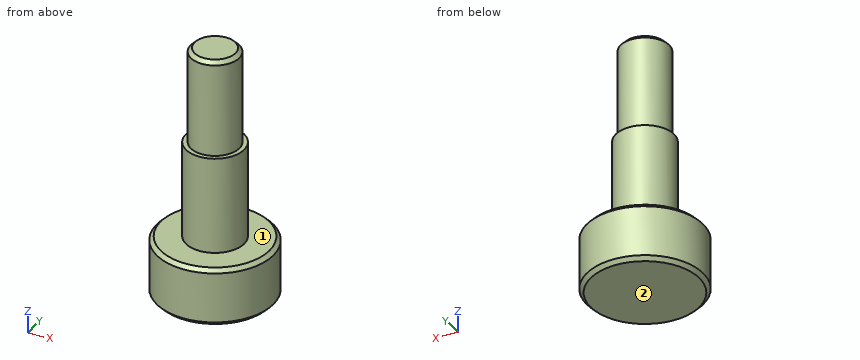
```python
from build123d import *

# Parameters (mm, degrees)
SKETCH_1_R      = 3
EXTRUDE_1_DEPTH = 3
SKETCH_2_R      = 1.5
EXTRUDE_2_DEPTH = 5
SKETCH_3_R      = 1.25
EXTRUDE_3_DEPTH = 5
CHAMFER_1_SIZE  = 0.2


with BuildPart() as part:
    # 草图1 → 凸台-拉伸1 (new body)
    with BuildSketch(Plane.XY):
        Circle(SKETCH_1_R)
    extrude(amount=EXTRUDE_1_DEPTH)

    # 草图2 → 凸台-拉伸2 (add)
    with BuildSketch(Plane.XY.offset(3)):
        Circle(SKETCH_2_R)
    extrude(amount=EXTRUDE_2_DEPTH)

    # 草图3 → 凸台-拉伸3 (add)
    with BuildSketch(Plane.XY.offset(8)):
        Circle(SKETCH_3_R)
    extrude(amount=EXTRUDE_3_DEPTH)

    # 倒角1
    chamfer_1_edges = [part.edges().sort_by_distance(p)[0] for p in [
        (-1.25, 0, 13),
        (-3, 0, 0),
        (-3, 0, 3),
    ]]
    chamfer(chamfer_1_edges, length=CHAMFER_1_SIZE)


solid = part.part
```
Input: part model. Units: mm. Frame: model coordinates. Face numbers are marked on the shaded views. A direction names the side the tool comes from. Give positions to 0.01 mm unless a question says otherwise; leave off trailing zeros. Order: outer loops, then holes, each group sorted by start corner. A loop starts at its lowest first (then second) coordinate and runs counter-clockwise, first axis right, second up.
1. Set-up query: the marked faces 1 and 2. Return all of +Z, -Z, +X, -X, +Y, -Y with unobstructed straight access to the full face (end or side cutting, diameter ignored); none if empty.
Computed:
face 1: +Z
face 2: -Z, +X, -X, +Y, -Y
2. Line query: probe 1 along Z at (x, y) = (-1.7, 1.4); probe 2 along Z at (x, y) = (-0.4, -1.35); probe 3 along Y at (x, z) = (-0.05, 4.25). Output: solid intervals per line, ascending.
Computed:
probe 1: z = 0 to 3
probe 2: z = 0 to 8
probe 3: y = -1.5 to 1.5
3. Pin query (flat end, axial travel): pin 1 Ø3 at (x, z) = (1, 9) entering from -Y; pin 2 Ø1 at (x, y) = (-1, 2) entering from +Z; pin 3 Ø2 at (x, z) = (-2, 3.5) entering from -Y. Return the tip coordinate at first contact, or that it passes through.
Computed:
pin 1: stops at y = -1.5
pin 2: stops at z = 3
pin 3: stops at y = -2.71
4. Cut plane D-D (z = 10.75). Return loops of the section in (x, y), and give its area (3 significant figures).
Computed:
outline: circle Ø2.5 at (0, 0)
area: 4.91 mm2
5. Cut plane A-A (x = 0). Return loops of the section in (y, z), and give its area (3 significant figures).
Computed:
outline: (-3, 0.2) - (-2.8, 0) - (2.8, 0) - (3, 0.2) - (3, 2.8) - (2.8, 3) - (1.5, 3) - (1.5, 8) - (1.25, 8) - (1.25, 12.8) - (1.05, 13) - (-1.05, 13) - (-1.25, 12.8) - (-1.25, 8) - (-1.5, 8) - (-1.5, 3) - (-2.8, 3) - (-3, 2.8) - close
area: 45.4 mm2
6. Cut plane C-C (z = 7.5). Return loops of the section in (x, y).
Computed:
outline: circle Ø3 at (0, 0)
